Can you work these out from the model? Positions are in its coordinate system, mm. A direction names the side the tool comes from. Coordinates: 2 decimals unless noted, no trailing zeros. Order: outer loops, then holes, each group sorted by start corner. A loop starts at its lowest first (then second) coordinate and runs counter-clockwise, first axis right, second up. Notation, with made-up numbers: (55.5, -17.75) -> (111.5, -17.75) arc R34 ccw to (111.5, 21.25) -> close; hole circle Ø3 at (15, -14.75). An arc over 180 degrees is marked (long way). Answer in a Markdown table with one row per item. Add a question column.
1. Imagine slicing it at C-C on x = 0. Write out the boundary of the cut face in (y, z), plus the area to 3 significant figures.
2. Imagine slicing it at D-D on z = -2.25. Write out the boundary of the cut face in (x, y).
3. If I drill on line 1 along Y through (x, z) = (0.5, -0.25); line 2 along Z through (x, y) = (1, 1.75); line 3 along Z through (x, y) = (4.5, 6.25), over which ranges is the centre line in solid material (lowest first)? Write a range as [from, to].
4. Will these pins go through, and if not, where does the flat tip stop? pin 1 (5 mm diameter, centred on x = -3.5, y = 7.5, fed in from -Z); pin 2 (1.5 mm diameter, centred on x = -3, y = 5, fed in from +Z); pin 3 (4 mm diameter, centred on y = 8, z = -3, fed in from +X).
5. On a 3-axis mill with a long thin cutter (end or side, diameter ignored), from which of +Z, -Z, +X, -X, +Y, -Y can I reach the whole of each face in a straight line? I mean faces 4 (the face through (-1.5, 2.46, 0.07)), 5 (the face through (4.164, 4.93, 0.009)). Say none if no direction works.
6. We'd pull the mould along Z, two halves only. Please class faces 1 (the face through (1.965, 4.93, -4.706)), 2 (the face through (4.706, 4.93, 1.965)), 3 (the face through (2.94, 4.93, 2.95)): pulls with the +Z half, pulls with the -Z half, needs draft (parallel to the pull), parting line crosses it, or undercut.
from build123d import *

# Parameters (mm, degrees)
BOSS_EXTRUDE1_DEPTH = 10
SKETCH2_R           = 1.5
CUT_EXTRUDE1_DEPTH  = 5


with BuildPart() as part:
    # Sketch1 → Boss-Extrude1 (new body)
    with BuildSketch(Plane(origin=(0, 0, 0), x_dir=(1, 0, 0), z_dir=(0, 1, 0))):
        with BuildLine():
            Line((-0.570751275, 4.458354836), (-0.96142982, 5.008557946))
            ThreePointArc((-0.96142982, 5.008557946), (-1.951685505, 4.711785616), (-2.861751742, 4.221418833))
            Line((-2.861751742, 4.221418833), (-2.748950841, 3.556115034))
            ThreePointArc((-2.748950841, 3.556115034), (-2.944126667, 2.944126667), (-3.556115034, 2.748950841))
            Line((-3.556115034, 2.748950841), (-4.221418833, 2.861751742))
            ThreePointArc((-4.221418833, 2.861751742), (-4.711785616, 1.951685505), (-5.008557946, 0.96142982))
            Line((-5.008557946, 0.96142982), (-4.458354836, 0.570751275))
            ThreePointArc((-4.458354836, 0.570751275), (-4.163623861, 0), (-4.458354836, -0.570751275))
            Line((-4.458354836, -0.570751275), (-5.008557946, -0.96142982))
            ThreePointArc((-5.008557946, -0.96142982), (-4.711785616, -1.951685505), (-4.221418833, -2.861751742))
            Line((-4.221418833, -2.861751742), (-3.556115034, -2.748950841))
            ThreePointArc((-3.556115034, -2.748950841), (-2.944126667, -2.944126667), (-2.748950841, -3.556115034))
            Line((-2.748950841, -3.556115034), (-2.861751742, -4.221418833))
            ThreePointArc((-2.861751742, -4.221418833), (-1.951685505, -4.711785616), (-0.96142982, -5.008557946))
            Line((-0.96142982, -5.008557946), (-0.570751275, -4.458354836))
            ThreePointArc((-0.570751275, -4.458354836), (0, -4.163623861), (0.570751275, -4.458354836))
            Line((0.570751275, -4.458354836), (0.96142982, -5.008557946))
            ThreePointArc((0.96142982, -5.008557946), (1.951685505, -4.711785616), (2.861751742, -4.221418833))
            Line((2.861751742, -4.221418833), (2.748950841, -3.556115034))
            ThreePointArc((2.748950841, -3.556115034), (2.944126667, -2.944126667), (3.556115034, -2.748950841))
            Line((3.556115034, -2.748950841), (4.221418833, -2.861751742))
            ThreePointArc((4.221418833, -2.861751742), (4.711785616, -1.951685505), (5.008557946, -0.96142982))
            Line((5.008557946, -0.96142982), (4.458354836, -0.570751275))
            ThreePointArc((4.458354836, -0.570751275), (4.163623861, 0), (4.458354836, 0.570751275))
            Line((4.458354836, 0.570751275), (5.008557946, 0.96142982))
            ThreePointArc((5.008557946, 0.96142982), (4.711785616, 1.951685505), (4.221418833, 2.861751742))
            Line((4.221418833, 2.861751742), (3.556115034, 2.748950841))
            ThreePointArc((3.556115034, 2.748950841), (2.944126667, 2.944126667), (2.748950841, 3.556115034))
            Line((2.748950841, 3.556115034), (2.861751742, 4.221418833))
            ThreePointArc((2.861751742, 4.221418833), (1.951685505, 4.711785616), (0.96142982, 5.008557946))
            Line((0.96142982, 5.008557946), (0.570751275, 4.458354836))
            ThreePointArc((0.570751275, 4.458354836), (0, 4.163623861), (-0.570751275, 4.458354836))
        make_face()
    extrude(amount=BOSS_EXTRUDE1_DEPTH)

    # Sketch2 → Cut-Extrude1 (cut)
    with BuildSketch(Plane.XZ):
        Circle(SKETCH2_R)
    extrude(amount=-CUT_EXTRUDE1_DEPTH, mode=Mode.SUBTRACT)


solid = part.part
Answers follow:
| question | item | result |
|---|---|---|
| 1 | outline | (0, -4.16) -> (10, -4.16) -> (10, 4.16) -> (0, 4.16) -> (0, 1.5) -> (5, 1.5) -> (5, -1.5) -> (0, -1.5) -> close |
| 1 | area | 68.3 mm² |
| 2 | outline | (-4.58, 0) -> (4.58, 0) -> (4.58, 10) -> (-4.58, 10) -> close |
| 3 | line 1 | y = [5, 10] |
| 3 | line 2 | z = [-5, -1.12], [1.12, 5] |
| 3 | line 3 | z = [-2.4, -0.6], [0.6, 2.4] |
| 4 | pin 1 | stops at z = -5 |
| 4 | pin 2 | stops at z = 4.58 |
| 4 | pin 3 | stops at x = 5 |
| 5 | face 4 | -Y |
| 5 | face 5 | +X, +Y, -Y |
| 6 | face 1 | pulls with the -Z half |
| 6 | face 2 | pulls with the +Z half |
| 6 | face 3 | undercut |
